Geometry check sheet. Reference: the model listing, model coordinates, mm. Face numbers are marked on the shaded views. Coordinates: 2 decimals unless noted, no trailing zeros. Order: outer loops, then holes, each group sorted by start corner. A loop starts at its lowest first (then second) coordinate and runs counter-clockwise, first axis right, second up. Notation, with made-up numbers: (76.25, 51.5) - (129.25, 51.5) arc R34 cw to (129.25, 82.5) - close; hole circle Ø4 at (63.5, -14). An arc over 180 degrees is marked (long way). Use CSV: the item, a comma, the result in double quotes. Start each with the question number.
1) Sectioned sample at A-A, the plane y = 34.5. Record the cut outline in (x, z).
2) Depth check by flat-ended pin: P1, Ø7.5, axis at x = 10, z = 35, coming from the +Y side; P2, Ø2, axis at x = 199, z = 12, coming from the +Y side. Enter the tip coordinate at first touch or a pass-through.
3) Thickness scan on probe 1 along Y at (x, z) = (104, 8); probe 2 along Z at (x, y) = (217.5, 20.5); probe 3 along Z at (x, y) = (148, 6). Record the ranges inside material, lowest first. Write a range as [from, to].
4) Draft check along Z on the marked faces 1, 2 and 3. Enter one of: released by +Z, released by -Z, zero draft, split by the parting line, or undercut.
5) Sectioned sample at B-B, the plane z = 53. Record the cut outline in (x, y), and give its area (3 significant figures).
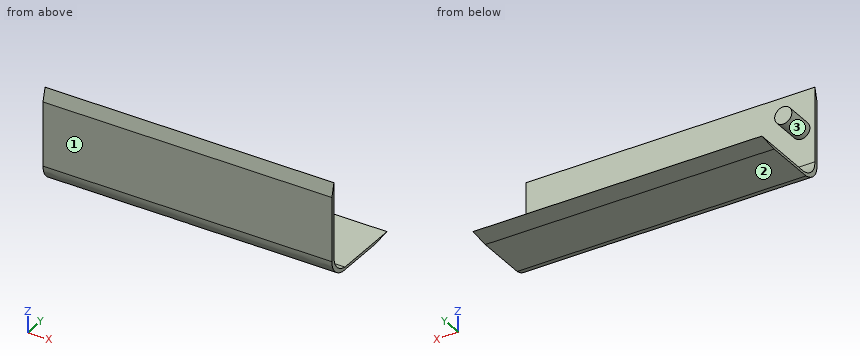
from build123d import *

# Parameters (mm, degrees)
F1_DEPTH = 254
F2_R     = 7.5365841045
F3_DEPTH = 25.4


# Not quite as in the source:
# - the program builds the solid bodies; features that only make, move or delete a surface that nothing else refers to are left out


with BuildPart() as f1:
    # F0 (on Right) → F1 (new body)
    with BuildSketch(Plane.YZ):
        with BuildLine():
            Line((2.9371477504, 67.7488154993), (0, 56.3350282609))
            Line((0, 56.3350282609), (0, 0))
            add(Edge.make_bspline(
                [(0, 0), (0, -8.9850798249), (6.8457759917, -15.2603751048), (15.4029959813, -16.6865773499)],
                knots=[0, 0, 0, 0, 22.7089002123, 22.7089002123, 22.7089002123, 22.7089002123], degree=3))
            Line((15.4029959813, -16.6865773499), (60.1857788861, -16.6865773499))
            Line((60.1857788861, -16.6865773499), (77.3849593316, -14.4004908129))
            Line((77.3849593316, -14.4004908129), (18.3401437317, -14.4004908129))
            add(Edge.make_bspline(
                [(2.9371477504, 2.286086537), (2.9371477504, -6.6989932879), (9.7829237421, -12.9742885678), (18.3401437317, -14.4004908129)],
                knots=[0, 0, 0, 0, 22.7089002123, 22.7089002123, 22.7089002123, 22.7089002123], degree=3))
            Line((2.9371477504, 2.286086537), (2.9371477504, 67.7488154993))
        make_face()
    extrude(amount=F1_DEPTH)

    # F2 (on face) → F3 (join)
    with BuildSketch(Plane(origin=(0, 2.9371477504, 0), x_dir=(-1, 0, 0), z_dir=(0, 1, 0))):
        with Locations((-11.9260810316, 33.5152037442)):
            Circle(F2_R)
    extrude(amount=F3_DEPTH)


solid = f1.part
Evaluation:
1,outline,"(0, -16.69) - (254, -16.69) - (254, -14.4) - (0, -14.4) - close"
2,P1,"y = 28.34"
2,P2,"y = 2.94"
3,probe 1,"[0, 2.94]"
3,probe 2,"[-16.69, -14.4]"
3,probe 3,"[-12.56, -7.2]"
4,face 1,"zero draft"
4,face 2,"released by -Z"
4,face 3,"undercut"
5,outline,"(0, 0) - (254, 0) - (254, 2.94) - (0, 2.94) - close"
5,area,"746 mm²"
